```python
from build123d import *

# Parameters (mm, degrees)
SKETCH_1_R          = 34
EXTRUDE_1_DEPTH     = 13.6
SKETCH_2_R          = 16.5
EXTRUDE_2_DEPTH     = 8.9
FILLET_1_R          = 1
SKETCH_3_R          = 4
CUT_EXTRUDE_1_DEPTH = 54.087192429
SKETCH_4_R          = 7.5
CUT_EXTRUDE_2_DEPTH = 54.087192429
M3X0_52_D           = 2.5
M3X0_53_D           = 2.5
SKETCH_15_R         = 20.204336051
CUT_EXTRUDE_3_DEPTH = 8.9


with BuildPart() as part:
    # Эскиз1 → Бобышка-Вытянуть1 (new body)
    with BuildSketch(Plane.XY):
        Circle(SKETCH_1_R)
    extrude(amount=EXTRUDE_1_DEPTH)

    # Эскиз2 → Бобышка-Вытянуть2 (add)
    with BuildSketch(Plane.XY.offset(13.6)):
        Circle(SKETCH_2_R)
    extrude(amount=EXTRUDE_2_DEPTH)

    # Скругление1
    fillet_1_edges = [part.edges().sort_by_distance(p)[0] for p in [
        (-16.5, 0, 22.5),
    ]]
    fillet(fillet_1_edges, radius=FILLET_1_R)

    # Эскиз3 → Вырез-Вытянуть1 (cut, through all)
    with BuildSketch(Plane(origin=(0, 0, 0), x_dir=(-1, 0, 0), z_dir=(0, 0, -1))):
        Circle(SKETCH_3_R)
    extrude(amount=-CUT_EXTRUDE_1_DEPTH, mode=Mode.SUBTRACT)

    # Эскиз4 → Вырез-Вытянуть2 (cut, through all)
    with BuildSketch(Plane.XY.offset(22.5)):
        Circle(SKETCH_4_R)
    extrude(amount=-CUT_EXTRUDE_2_DEPTH, mode=Mode.SUBTRACT)

    # Отверстие обработанное метчиком M3x0.52 (through all)
    with Locations(Plane(origin=(5.176865527, -11.054831177, 0), x_dir=(1, 0, 0), z_dir=(0, 0, -1))):
        with Locations((-11.426865527, -21.880148725), (-11.426865527, -0.22951363), (7.323134473, -11.054831177)):
            Hole(M3X0_52_D / 2)

    # Отверстие обработанное метчиком M3x0.53 (through all)
    with Locations(Plane(origin=(7.745995854, 28.191062488, 0), x_dir=(1, 0, 0), z_dir=(0, 0, -1))):
        with Locations((6.004004146, 4.375363884), (-35.245995854, 28.191062488), (6.004004146, 52.006761092)):
            Hole(M3X0_53_D / 2)

    # Эскиз15 → Вырез-Вытянуть3 (cut)
    with BuildSketch(Plane.XY.offset(22.5)):
        Circle(SKETCH_15_R)
    extrude(amount=-CUT_EXTRUDE_3_DEPTH, mode=Mode.SUBTRACT)


solid = part.part
```
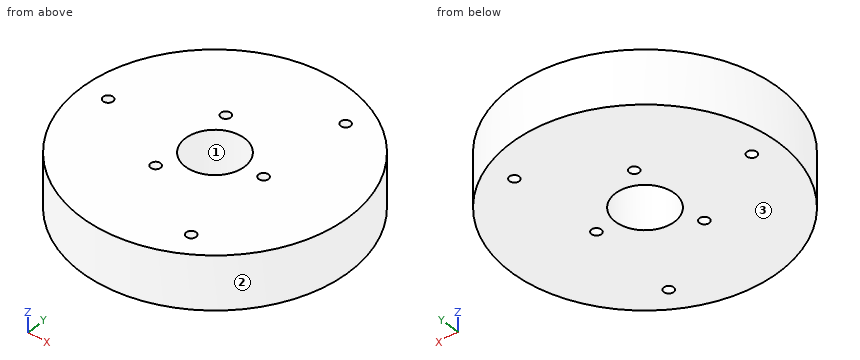
Input: part model. Units: mm. Frame: model coordinates. Face numbers are marked on the shaded views. Coordinates: 2 decimals unless noted, no trailing zeros. Loops run counter-clockwise (first coordinate to the right, second up) from the corner with the lowest first, then second, coordinate; pieces in that order, holes last. Notation, with made-up numbers: M 41.5,-32 L 72.5,-32 A27 cw 72.5,-10 Z; hole C 50.25,-16.75 d5. An arc over 180 degrees is marked long. One line per item, written item: value.
(1) Line query: line 1 along Y through (x, z) = (-6.25, 3); line 2 along Y through (x, z) = (-0.5, 6.5); line 3 along Y through (x, z) = (13.5, 7.25). Output: solid intervals per line, ascending. Write a range as from..to.
Filled in:
line 1: -33.42..-12.08, -9.58..-4.15, 4.15..9.58, 12.08..33.42
line 2: -34..-7.48, 7.48..34
line 3: -31.2..-25.04, -22.59..-0.75, 0.75..22.59, 25.04..31.2
(2) Section D-D (x = -27.5). Output: boundary loops of the cut face in (y, z).
Filled in:
outline: M -19.99,0 L -1.25,0 L -1.25,13.6 L -19.99,13.6 Z; M 1.25,0 L 19.99,0 L 19.99,13.6 L 1.25,13.6 Z
(3) Pull-direction query (Y, two-part tool) for the marked faces 1, 2 and 3; classes: +Y half, -Y half, draft (parallel to the pull), parting line (faces both ways), or undercut.
Filled in:
face 1: undercut
face 2: parting line
face 3: draft
(4) Pin query (flat end, axial travel): pin 1 (1 mm diameter, centred on x = 6, z = 5, fed in from +Y); pin 2 (3 mm diameter, centred on x = 10.5, z = 7.5, fed in from +Y); pin 3 (4 mm diameter, centred on x = -14.5, z = 2, fed in from -Y). Return the tip coordinate at first contact, or that it passes through.
Filled in:
pin 1: y = 33.55
pin 2: y = 32.79
pin 3: y = -31.62
(5) Section A-A (x = 0). Output: boundary loops of the cut face in (y, z), and give its area (3 significant figures).
Filled in:
outline: M -34,0 L -7.5,0 L -7.5,13.6 L -34,13.6 Z; M 7.5,0 L 34,0 L 34,13.6 L 7.5,13.6 Z
area: 721 mm^2
(6) Section C-C (z = 2.5). Output: boundary loops of the cut face in (x, y).
Filled in:
outline: C 0,0 d68; hole C -27.5,0 d2.5; hole C -6.25,-10.83 d2.5; hole C 0,0 d15; hole C -6.25,10.83 d2.5; hole C 12.5,0 d2.5; hole C 13.75,-23.82 d2.5; hole C 13.75,23.82 d2.5
(7) Section B-B (y = 0). Output: boundary loops of the cut face in (x, z), and give its area (3 significant figures).
Filled in:
outline: M -34,0 L -28.75,0 L -28.75,13.6 L -34,13.6 Z; M -26.25,0 L -7.5,0 L -7.5,13.6 L -26.25,13.6 Z; M 7.5,0 L 11.25,0 L 11.25,13.6 L 7.5,13.6 Z; M 13.75,0 L 34,0 L 34,13.6 L 13.75,13.6 Z
area: 653 mm^2
